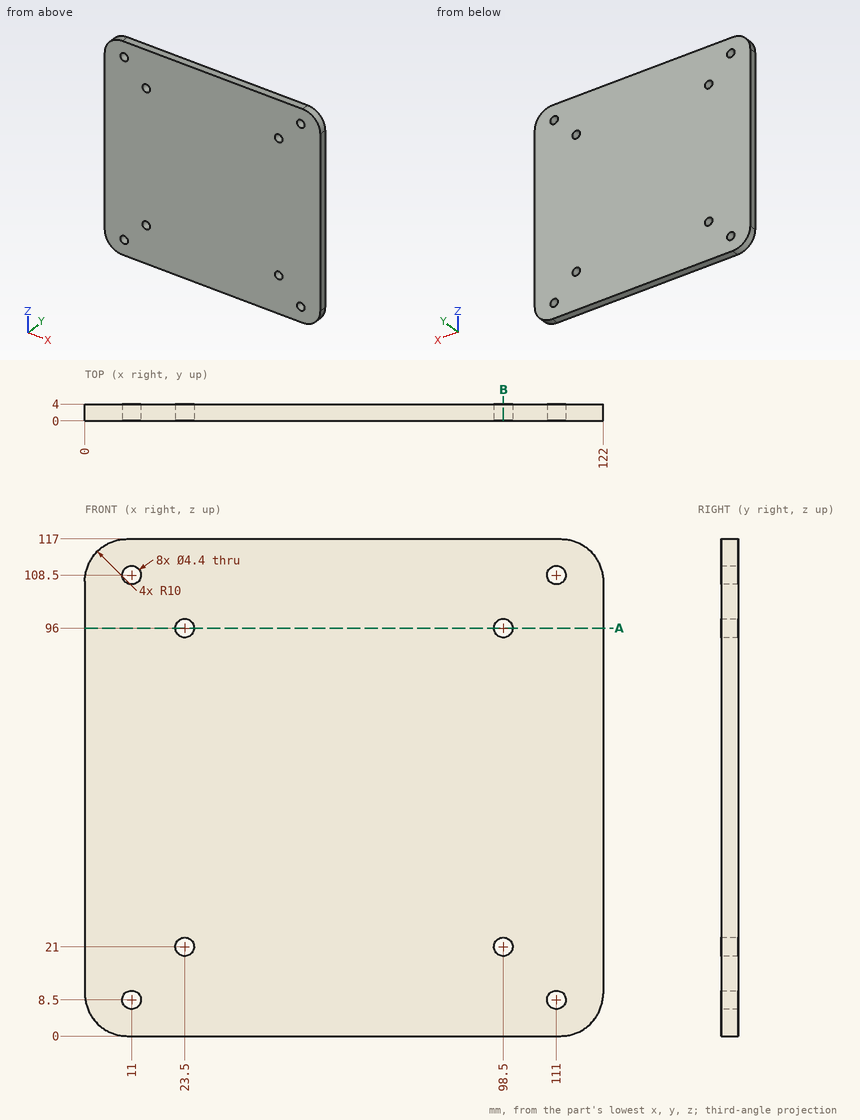
Drawing for the job (mm, zero at the part's lowest x, y, z). Round coordinates to 2 decimals unless told otherwise and drop trailing zeros. Loops run counter-clockwise (first coordinate to the right, second up) from the corner with the lowest first, then second, coordinate; pieces in that order, holes last. Notation, with made-up numbers: (5, -5) - (34, -5) arc R19 ccw to (34, 25) - close; hole circle Ø7 at (60, 61.25). An arc over 180 degrees is marked (long way). Write each question's results on one line, items separated by ' | '.
(1) Saw through at B-B, the plane x = 98.5. List the corners of the cut face in (y, z).
Answer below:
outline: (0, 0) - (4, 0) - (4, 18.8) - (0, 18.8) - close; (0, 23.2) - (4, 23.2) - (4, 93.8) - (0, 93.8) - close; (0, 98.2) - (4, 98.2) - (4, 117) - (0, 117) - close
(2) Wall check: L1, parallel to X at y = 1.8, z = 96; L2, parallel to X at y = 1.6, z = 8.5; L3, parallel to Z at x = 112.5, y = 1.15. Give the ranges that are in metal, low to high.
Answer below:
L1: x = 0 to 21.3, 25.7 to 96.3, 100.7 to 122 | L2: x = 0.11 to 8.8, 13.2 to 108.8, 113.2 to 121.89 | L3: z = 0.01 to 6.89, 10.11 to 106.89, 110.11 to 116.99
(3) Saw through at A-A, the plane z = 96. List the corners of the cut face in (x, y), then the cut area to 3 significant figures.
Answer below:
outline: (0, 0) - (21.3, 0) - (21.3, 4) - (0, 4) - close; (25.7, 0) - (96.3, 0) - (96.3, 4) - (25.7, 4) - close; (100.7, 0) - (122, 0) - (122, 4) - (100.7, 4) - close | area: 453 mm^2
